Here's how the part is built. I have some questions about the finished solid (model axes, mm). Face numbers are marked on the shaded views. A direction names the side the tool comes from. Coordinates: 2 decimals unless noted, no trailing zeros. Write each loop counter-clockwise with the first axis right and the second up, starting at its lowest first coordinate (ties: lowest second). Pieces come first, ordered by that corner, then holes.
Item 1: I want a section at B-B (z = 0). Please give me the cut outline in (x, y).
Item 2: Please list where these lines run through material, in increasing order: line 1 (X direction, y = 21.5, z = 40); line 2 (X direction, y = -3, z = 12.5); line 3 (Y direction, x = 28, z = 43.5).
Item 3: I want a section at D-D (z = -12.5). Please give me the cut outline in (x, y), and give its area (3 significant figures).
Item 4: I'm going to push flat-ended pins straight in: P1, Ø1, axis at x = 0, z = 3.5, coming from the +Y side; P2, Ø2.5, axis at x = -17, z = 13.5, coming from the -Y side; P3, Ø8, axis at x = 13, y = -26, coming from the -Z side. Where does each tip first touch, or does it pass through?
Item 5: I want a section at C-C (z = 53.5). Please give me the cut outline in (x, y), and give its area (3 significant figures).
Item 6: For the marked faces 1, 2 and 3, which set-ups out of +Z, -Z, +X, -X, +Y, -Y let a thin tool reach every point of the face, with its end or its side?
Item 7: I want a section at A-A (y = 17.5). Count the separate pieces of the cut face and the enclosed holes in it, and give its area (3 significant figures).
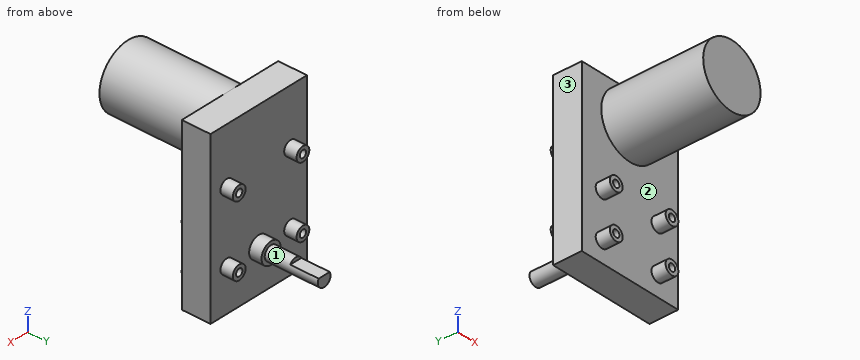
from build123d import *

# Parameters (mm, degrees)
SKETCH_1_W          = 60.5
SKETCH_1_H          = 95.5
EXTRUDE_1_DEPTH     = 16.2
SKETCH_2_R          = 6
SKETCH_2_R_2        = 4
SKETCH_2_R_3        = 2
EXTRUDE_2_DEPTH     = 7
SKETCH_3_R          = 4
EXTRUDE_3_DEPTH     = 30
CUT_EXTRUDE_START   = -16
CUT_EXTRUDE_1_DEPTH = 16
SKETCH_5_R          = 4
SKETCH_5_R_2        = 2
EXTRUDE_4_DEPTH     = 8
SKETCH_6_R          = 18
EXTRUDE_5_DEPTH     = 57.6


with BuildPart() as part:
    # 草图1 → 凸台-拉伸1 (new body)
    with BuildSketch(Plane(origin=(0, 0, 0), x_dir=(1, 0, 0), z_dir=(0, 1, 0))):
        with Locations((0, -23.75)):
            Rectangle(SKETCH_1_W, SKETCH_1_H)
    extrude(amount=EXTRUDE_1_DEPTH)

    # 草图2 → 凸台-拉伸2 (add)
    # profile 1 of 5: a face of its own
    with BuildSketch(Plane(origin=(0, 16.2, 0), x_dir=(1, 0, 0), z_dir=(0, 1, 0))):
        with Locations(Location((0, 0, 0), (0, 0, 90))):
            Circle(SKETCH_2_R)
    # profile 2 of 5: a face of its own
    with BuildSketch(Plane(origin=(0, 16.2, 0), x_dir=(1, 0, 0), z_dir=(0, 1, 0))):
        with Locations(Location((-20, 0, 0), (0, 0, 90))):
            Circle(SKETCH_2_R_2)
        with Locations(Location((-20, 0, 0), (0, 0, 270))):
            Circle(SKETCH_2_R_3, mode=Mode.SUBTRACT)
    # profile 3 of 5: a face of its own
    with BuildSketch(Plane(origin=(0, 16.2, 0), x_dir=(1, 0, 0), z_dir=(0, 1, 0))):
        with Locations(Location((20, 0, 0), (0, 0, 90))):
            Circle(SKETCH_2_R_2)
        with Locations(Location((20, 0, 0), (0, 0, 270))):
            Circle(SKETCH_2_R_3, mode=Mode.SUBTRACT)
    # profile 4 of 5: a face of its own
    with BuildSketch(Plane(origin=(0, 16.2, 0), x_dir=(1, 0, 0), z_dir=(0, 1, 0))):
        with Locations(Location((20, -40, 0), (0, 0, 90))):
            Circle(SKETCH_2_R_2)
        with Locations(Location((20, -40, 0), (0, 0, 270))):
            Circle(SKETCH_2_R_3, mode=Mode.SUBTRACT)
    # profile 5 of 5: a face of its own
    with BuildSketch(Plane(origin=(0, 16.2, 0), x_dir=(1, 0, 0), z_dir=(0, 1, 0))):
        with Locations(Location((-20, -40, 0), (0, 0, 90))):
            Circle(SKETCH_2_R_2)
        with Locations(Location((-20, -40, 0), (0, 0, 270))):
            Circle(SKETCH_2_R_3, mode=Mode.SUBTRACT)
    extrude(amount=EXTRUDE_2_DEPTH)

    # 草图3 → 凸台-拉伸3 (add)
    with BuildSketch(Plane(origin=(0, 23.2, 0), x_dir=(1, 0, 0), z_dir=(0, 1, 0))):
        with Locations(Location((0, 0, 0), (0, 0, 270))):
            Circle(SKETCH_3_R)
    extrude(amount=EXTRUDE_3_DEPTH)

    # 草图4 → 切除-拉伸1 (cut)
    with BuildSketch(Plane(origin=(0, 53.2, 0), x_dir=(1, 0, 0), z_dir=(0, 1, 0)).offset(CUT_EXTRUDE_START)):
        with BuildLine():
            Line((-3.464101615, -2), (3.464101615, -2))
            ThreePointArc((3.464101615, -2), (0, -4), (-3.464101615, -2))
        make_face()
    extrude(amount=CUT_EXTRUDE_1_DEPTH, mode=Mode.SUBTRACT)

    # 草图5 → 凸台-拉伸4 (add)
    # profile 1 of 4: a face of its own
    with BuildSketch(Plane(origin=(0, 0, 0), x_dir=(-1, 0, 0), z_dir=(0, -1, 0))):
        with Locations(Location((-17.5, 12.5, 0), (0, 0, 90))):
            Circle(SKETCH_5_R)
        with Locations(Location((-17.5, 12.5, 0), (0, 0, 90))):
            Circle(SKETCH_5_R_2, mode=Mode.SUBTRACT)
    # profile 2 of 4: a face of its own
    with BuildSketch(Plane(origin=(0, 0, 0), x_dir=(-1, 0, 0), z_dir=(0, -1, 0))):
        with Locations(Location((17.5, 12.5, 0), (0, 0, 90))):
            Circle(SKETCH_5_R)
        with Locations(Location((17.5, 12.5, 0), (0, 0, 90))):
            Circle(SKETCH_5_R_2, mode=Mode.SUBTRACT)
    # profile 3 of 4: a face of its own
    with BuildSketch(Plane(origin=(0, 0, 0), x_dir=(-1, 0, 0), z_dir=(0, -1, 0))):
        with Locations(Location((17.5, -12.5, 0), (0, 0, 90))):
            Circle(SKETCH_5_R)
        with Locations(Location((17.5, -12.5, 0), (0, 0, 90))):
            Circle(SKETCH_5_R_2, mode=Mode.SUBTRACT)
    # profile 4 of 4: a face of its own
    with BuildSketch(Plane(origin=(0, 0, 0), x_dir=(-1, 0, 0), z_dir=(0, -1, 0))):
        with Locations(Location((-17.5, -12.5, 0), (0, 0, 90))):
            Circle(SKETCH_5_R)
        with Locations(Location((-17.5, -12.5, 0), (0, 0, 90))):
            Circle(SKETCH_5_R_2, mode=Mode.SUBTRACT)
    extrude(amount=EXTRUDE_4_DEPTH)

    # 草图6 → 凸台-拉伸5 (add)
    with BuildSketch(Plane.XZ):
        with Locations(Location((0, 53.5, 0), (0, 0, 90))):
            Circle(SKETCH_6_R)
    extrude(amount=EXTRUDE_5_DEPTH)


solid = part.part
Answer:
1. outline: (-30.25, 0) - (30.25, 0) - (30.25, 16.2) - (24, 16.2) - (24, 23.2) - (22, 23.2) - (22, 16.2) - (18, 16.2) - (18, 23.2) - (16, 23.2) - (16, 16.2) - (6, 16.2) - (6, 23.2) - (4, 23.2) - (4, 53.2) - (-4, 53.2) - (-4, 23.2) - (-6, 23.2) - (-6, 16.2) - (-16, 16.2) - (-16, 23.2) - (-18, 23.2) - (-18, 16.2) - (-22, 16.2) - (-22, 23.2) - (-24, 23.2) - (-24, 16.2) - (-30.25, 16.2) - close
2. line 1: x = -24 to -22, -18 to -16, 16 to 18, 22 to 24
2. line 2: x = -21.5 to -19.5, -15.5 to -13.5, 13.5 to 15.5, 19.5 to 21.5
2. line 3: y = 0 to 16.2
3. outline: (-30.25, 0) - (-21.5, 0) - (-21.5, -8) - (-19.5, -8) - (-19.5, 0) - (-15.5, 0) - (-15.5, -8) - (-13.5, -8) - (-13.5, 0) - (13.5, 0) - (13.5, -8) - (15.5, -8) - (15.5, 0) - (19.5, 0) - (19.5, -8) - (21.5, -8) - (21.5, 0) - (30.25, 0) - (30.25, 16.2) - (-30.25, 16.2) - close
3. area: 1,040 mm2
4. P1: stops at y = 37.2
4. P2: stops at y = -8
4. P3: stops at z = 37.91
5. outline: (-30.25, 0) - (-18, 0) - (-18, -57.6) - (18, -57.6) - (18, 0) - (30.25, 0) - (30.25, 16.2) - (-30.25, 16.2) - close
5. area: 3,050 mm2
6. face 1: +Y
6. face 2: -Y
6. face 3: +Z, -Z, -X, +Y, -Y
7. separate pieces: 5
7. enclosed holes: 4
7. area: 264 mm2
